Work out the finished part from the listing and answer in its coordinate system (mm). A direction names the side the tool comes from. Give positions to 0.01 mm unless a question says otherwise; leave off trailing zeros. Write each loop counter-clockwise with the first axis right and the second up, starting at its lowest first coordinate (ties: lowest second). Pieces come first, ordered by that corner, then holes.
1) Determine the mould class of faces 1 (the face through (45, 64.919, 3)), 2 (the face through (-11.068, 7, 3)), 3 (the face through (88.142, 7, 2)), 4 (the face through (90, 8, 4.775)) for opening direction X: pulls with the +X half, pulls with the -X half, needs draft (parallel to the pull), parting line crosses it, or undercut.
2) Find section C-C (z = 3.5). Determine the outline of the cut face in (x, y).
3) Straight lines are drawn through the part: probe 1 along Y at (x, z) = (48, 3.75); probe 2 along X at (y, z) = (2, 3); probe 3 along X at (y, z) = (-30, 5.5). For each, find the intervals that lie inside material, in ascending order.
4) A tool of negligible diameter and unlimited length cuts with its end or side. For faces 5 (the face through (45, 50.494, 2)), 6 (the face through (103.232, 7, 3)), from which of +Z, -Z, +X, -X, +Y, -Y can it reach the whole face along a straight path? Write none if from no direction.
5) Given pin 1 Ø1 at (x, y) = (6.5, -4.5) entering from -Z, flat-ended and moving along its own axis, determine where the tip first touches the part or whether it passes through.
6) Find section A-A (x = 78.5). Determine the outline of the cut face in (y, z), plus the area to 3 significant figures.
7) Find section B-B (y = -2). Determine the outline of the cut face in (x, z), plus the area to 3 significant figures.
```python
from build123d import *

# Parameters (mm, degrees)
SKETCH1_W               = 114.3
SKETCH1_H               = 114.3
BOSS_EXTRUDE1_DEPTH     = 6.35
SKETCH2_W               = 100.12
SKETCH2_H               = 101.45
CUT_EXTRUDE1_DEPTH      = 1.5748
SKETCH4_W               = 84.12
SKETCH4_H               = 85.45
CUT_EXTRUDE3_DEPTH      = 2.5748
CUT_EXTRUDE3_DEPTH_BACK = 5.7752


with BuildPart() as part:
    # Sketch1 → Boss-Extrude1 (new body)
    with BuildSketch(Plane.XY):
        with Locations((46.081843575, 7.768994413)):
            Rectangle(SKETCH1_W, SKETCH1_H)
    extrude(amount=BOSS_EXTRUDE1_DEPTH)

    # Sketch2 → Cut-Extrude1 (cut)
    with BuildSketch(Plane.XY.offset(6.35)):
        with Locations((46.081843575, 7.768994413)):
            Rectangle(SKETCH2_W, SKETCH2_H)
    extrude(amount=-CUT_EXTRUDE1_DEPTH, mode=Mode.SUBTRACT)

    # Sketch4 → Cut-Extrude3 (cut, two sides)
    with BuildSketch(Plane.XY.offset(4.7752)) as cut_extrude3_sk:
        with Locations((46.081843575, 7.768994413)):
            Rectangle(SKETCH4_W, SKETCH4_H)
    extrude(amount=CUT_EXTRUDE3_DEPTH, mode=Mode.SUBTRACT)
    extrude(cut_extrude3_sk.sketch, amount=-CUT_EXTRUDE3_DEPTH_BACK, mode=Mode.SUBTRACT)


solid = part.part
```
Results:
1. face 1: needs draft
1. face 2: pulls with the -X half
1. face 3: undercut
1. face 4: undercut
2. outline: (-11.07, -49.38) - (103.23, -49.38) - (103.23, 64.92) - (-11.07, 64.92) - close; hole (4.02, -34.96) - (88.14, -34.96) - (88.14, 50.49) - (4.02, 50.49) - close
3. probe 1: y = -49.38 to -34.96, 50.49 to 64.92
3. probe 2: x = -11.07 to 4.02, 88.14 to 103.23
3. probe 3: x = -11.07 to -3.98, 96.14 to 103.23
4. face 5: +Z, -Z
4. face 6: +Z, -Z, +X, +Y, -Y
5. pin 1: passes through
6. outline: (-49.38, 0) - (-34.96, 0) - (-34.96, 4.78) - (-42.96, 4.78) - (-42.96, 6.35) - (-49.38, 6.35) - close; (50.49, 0) - (64.92, 0) - (64.92, 6.35) - (58.49, 6.35) - (58.49, 4.78) - (50.49, 4.78) - close
6. area: 158 mm2
7. outline: (-11.07, 0) - (4.02, 0) - (4.02, 4.78) - (-3.98, 4.78) - (-3.98, 6.35) - (-11.07, 6.35) - close; (88.14, 0) - (103.23, 0) - (103.23, 6.35) - (96.14, 6.35) - (96.14, 4.78) - (88.14, 4.78) - close
7. area: 166 mm2
